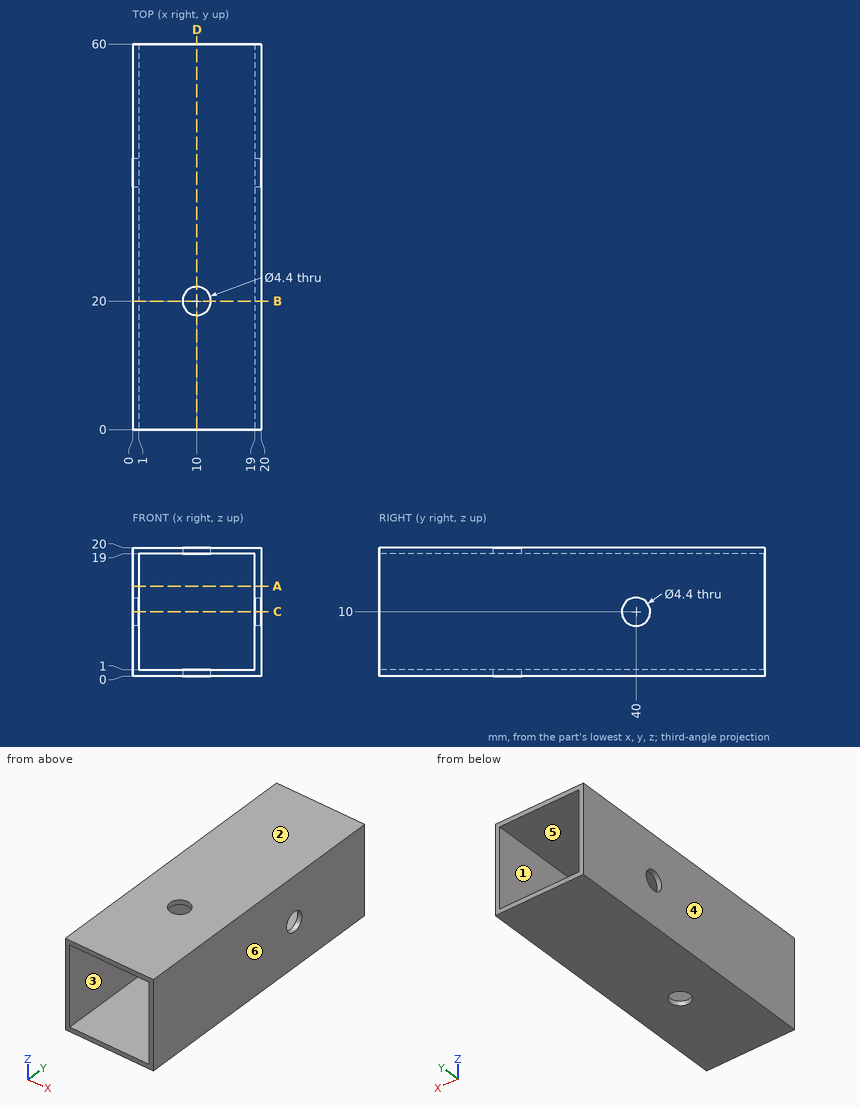
Part print with two shaded views. Sizes in mm from the minimum x, y, z corner. A direction names the side the tool comes from. Coordinates: 2 decimals unless noted, no trailing zeros. Write each loop counter-clockwise with the first axis right and the second up, starting at its lowest first coordinate (ties: lowest second). Pieces come first, ordered by that corner, then holes.
1. Pull direction X, two halves, no side cores. Call the marked faces 3, 4, 5 and 6: released by +X, released by -X, zero draft, split by the parting line, or undercut.
Answer block:
face 3: undercut
face 4: released by -X
face 5: undercut
face 6: released by +X
2. Band-saw the part on B-B, the plane y = 20. Give the cut face in (x, z).
Answer block:
outline: (0, 0) - (7.8, 0) - (7.8, 1) - (1, 1) - (1, 19) - (7.8, 19) - (7.8, 20) - (0, 20) - close; (12.2, 0) - (20, 0) - (20, 20) - (12.2, 20) - (12.2, 19) - (19, 19) - (19, 1) - (12.2, 1) - close
3. Drop a flat-ended pin along its axis: pin 1 (12 mm diameter, centred on x = 4, z = 7.5, fed in from -Y). Give the stop position or say it passes through.
Answer block:
pin 1: stops at y = 0
4. 3-axis set-ups, long thin cutter, end or side, ignore diameter. For the marked faces 1 and 2: which of +Z, -Z, +X, -X, +Y, -Y reach the whole face in a straight line?
Answer block:
face 1: +Y, -Y
face 2: +Z, +X, -X, +Y, -Y
5. Band-saw the part on A-A, the plane z = 14. Give the cut face in (x, y).
Answer block:
outline: (0, 0) - (1, 0) - (1, 60) - (0, 60) - close; (19, 0) - (20, 0) - (20, 60) - (19, 60) - close
6. Band-saw the part on C-C, the plane z = 10. Give the cut face in (x, y).
Answer block:
outline: (0, 0) - (1, 0) - (1, 37.8) - (0, 37.8) - close; (0, 42.2) - (1, 42.2) - (1, 60) - (0, 60) - close; (19, 0) - (20, 0) - (20, 37.8) - (19, 37.8) - close; (19, 42.2) - (20, 42.2) - (20, 60) - (19, 60) - close
7. Band-saw the part on D-D, the plane x = 10. Give the cut face in (y, z).
Answer block:
outline: (0, 0) - (17.8, 0) - (17.8, 1) - (0, 1) - close; (0, 19) - (17.8, 19) - (17.8, 20) - (0, 20) - close; (22.2, 0) - (60, 0) - (60, 1) - (22.2, 1) - close; (22.2, 19) - (60, 19) - (60, 20) - (22.2, 20) - close
8. Drill centre lines: probe 1 along Y at (x, z) = (10, 19.8); probe 2 along X at (y, z) = (16, 12.75); probe 3 along Z at (x, y) = (0.45, 40). Where is each one in solid material? Low to high.
Answer block:
probe 1: y = 0 to 17.8, 22.2 to 60
probe 2: x = 0 to 1, 19 to 20
probe 3: z = 0 to 7.8, 12.2 to 20
